Autodesk Inventor part; units mm, degrees
ref_plane "YZ Plane" through (0, 0, 0) normal (1, 0, 0) x (0, 1, 0)
ref_plane "XZ Plane" through (0, 0, 0) normal (0, 1, 0) x (-1, 0, 0)
ref_plane "XY Plane" through (0, 0, 0) normal (0, 0, 1) x (1, 0, 0)
sketch "スケッチ1" plane through (0, 0, 0) normal (0, 1, 0) x (-1, 0, 0)
  circle A0 centre (0, 0) radius 2
  circle A1 centre (0, 0) radius 3.2
  circle A2 centre (0, 0) radius 3.5 construction
  line L0 (3.5, 2.0207) -> (3.5, -2.0207)
  line L1 (3.5, -2.0207) -> (0, -4.0415)
  line L2 (0, -4.0415) -> (-3.5, -2.0207)
  line L3 (-3.5, -2.0207) -> (-3.5, 2.0207)
  line L4 (-3.5, 2.0207) -> (0, 4.0415)
  line L5 (0, 4.0415) -> (3.5, 2.0207)
  line L6 (0, 4.5564) -> (0, -4.4801) construction
  line L7 (3.3581, 0) -> (-3.3581, 0) construction
  point P0 (1.75, 3.0311)
  dimension "d2" = 7
  dimension "d0" = 6.4
  dimension "d1" = 4
extrude "押し出し1" add sketch "スケッチ1" along normal blind 0.6 contours A1 | L0 L1 L2 L3 L4 L5
extrude "押し出し2" add sketch "スケッチ1" against normal blind 1.3 contours A1
thread "ねじ1"
properties part number "SF419" material "鉄、ダクタイル鋳鉄"
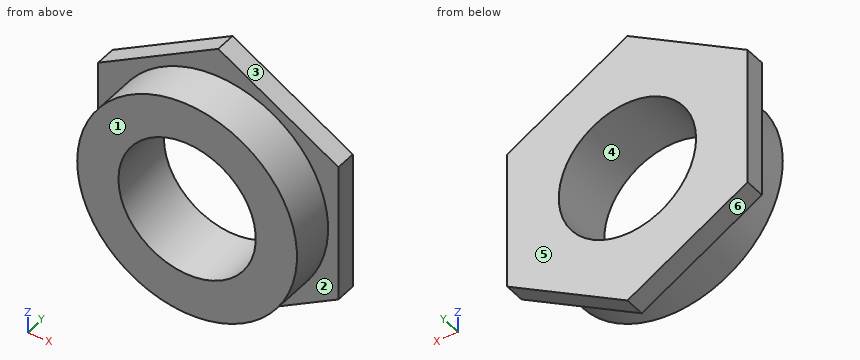
Verification items for the finished model (mm, model axes). Face numbers are marked on the shaded views. A direction names the side the tool comes from. Round coordinates to 2 decimals unless told otherwise and drop trailing zeros. Loops run counter-clockwise (first coordinate to the right, second up) from the corner with the lowest first, then second, coordinate; pieces in that order, holes last. Notation, with made-up numbers: (69.5, -37) - (123.5, -37) arc R36 ccw to (123.5, -1) - close; hole circle Ø7 at (-35.5, -39.75). An arc over 180 degrees is marked (long way). Use one line per item in the form item = value.
1. Scan lines: probe 1 along Z at (x, y) = (0, -0.25); probe 2 along Z at (x, y) = (-1.25, -0.9); probe 3 along Y at (x, z) = (3, 2). Record each from-to range of solid material in increasing order.
A:
probe_1 = -3.2 to -2, 2 to 3.2
probe_2 = -2.95 to -1.56, 1.56 to 2.95
probe_3 = 0 to 0.6
2. Draft check along X on the marked faces 3, 4, 5 and 6. Enter one of: pulls with the +X half, pulls with the -X half, needs draft (parallel to the pull), parting line crosses it, or undercut.
A:
face_3 = pulls with the +X half
face_4 = undercut
face_5 = needs draft
face_6 = pulls with the -X half
3. Section check D-D on z = -3. Record the cut outline in (x, y), and give its area (3 significant figures).
A:
outline = (-1.8, 0) - (-1.11, 0) - (-1.11, -1.3) - (1.11, -1.3) - (1.11, 0) - (1.8, 0) - (1.8, 0.6) - (-1.8, 0.6) - close
area = 5.06 mm²
4. Section check A-A on z = 0. Record the cut outline in (x, y), and give its area (3 significant figures).
A:
outline = (-3.5, 0) - (-3.2, 0) - (-3.2, -1.3) - (-2, -1.3) - (-2, 0.6) - (-3.5, 0.6) - close; (2, -1.3) - (3.2, -1.3) - (3.2, 0) - (3.5, 0) - (3.5, 0.6) - (2, 0.6) - close
area = 4.92 mm²
5. Section check C-C on x = 0.5. Record the cut outline in (y, z).
A:
outline = (-1.3, -3.16) - (0, -3.16) - (0, -3.75) - (0.6, -3.75) - (0.6, -1.94) - (-1.3, -1.94) - close; (-1.3, 1.94) - (0.6, 1.94) - (0.6, 3.75) - (0, 3.75) - (0, 3.16) - (-1.3, 3.16) - close
6. Access from +Z, -Z, +X, -X, +Y, -Y to the whole of each face (thin tool, end or side, straight path). Record for the marked faces 1 and 2.
A:
face_1 = +Z, -Z, +X, -X, -Y
face_2 = -Y
7. Section check B-B on y = 0.45. Record the cut outline in (x, z), and give its area (3 significant figures).
A:
outline = (-3.5, -2.02) - (0, -4.04) - (3.5, -2.02) - (3.5, 2.02) - (0, 4.04) - (-3.5, 2.02) - close; hole circle Ø4 at (0, 0)
area = 29.9 mm²
